Could you check a few things on this model? Use its own coordinates, in mm. Face numbers are marked on the shaded views. Give positions to 0.01 mm unless a question says otherwise; leave off trailing zeros. Order: outer loops, then holes, each group sorted by start corner. A loop starts at its lowest first (then second) coordinate and runs counter-clockwise, first axis right, second up. Notation, with made-up numbers: (82, 33) -> (109, 33) arc R21 ccw to (109, 53) -> close; hole circle Ø2 at (-30.75, -19). An arc over 180 degrees is marked (long way). One line per item, written item: value.
```python
from build123d import *

# Parameters (mm, degrees)
SKETCH1_W                      = 47.625
SKETCH1_H                      = 22.225
BOSS_EXTRUDE1_DEPTH            = 304.8
CUT_EXTRUDE1_REACH             = 27.4
SKETCH2_R                      = 14.2875
SKETCH2_R_2                    = 19.05
CUT_EXTRUDE1_DIRECTION_2_DEPTH = 1
CUT_EXTRUDE2_REACH             = 27.4
SKETCH3_R                      = 12.7
CUT_EXTRUDE2_DIRECTION_2_DEPTH = 1
SKETCH7_R                      = 4.7625
CUT_EXTRUDE3_DEPTH             = 24.8125
CUT_EXTRUDE3_DEPTH_BACK        = 2.5875
CUT_EXTRUDE4_REACH             = 27.4
SKETCH8_R                      = 3.3782
CUT_EXTRUDE4_DIRECTION_2_DEPTH = 1
CUT_EXTRUDE5_REACH             = 27.4
SKETCH9_R                      = 7.9375
CUT_EXTRUDE5_DIRECTION_2_DEPTH = 1
CUT_EXTRUDE6_REACH             = 27.4
SKETCH10_R                     = 1.5875
CUT_EXTRUDE6_DIRECTION_2_DEPTH = 1


with BuildPart() as part:
    # Sketch1 → Boss-Extrude1 (new body)
    with BuildSketch(Plane.XY):
        with BuildLine():
            Line((-23.8125, -12.7), (23.8125, -12.7))
            ThreePointArc((23.8125, -12.7), (24.935032015, -12.235032015), (25.4, -11.1125))
            Line((25.4, -11.1125), (25.4, 11.1125))
            ThreePointArc((25.4, 11.1125), (24.935032015, 12.235032015), (23.8125, 12.7))
            Line((23.8125, 12.7), (-23.8125, 12.7))
            ThreePointArc((-23.8125, 12.7), (-24.935032015, 12.235032015), (-25.4, 11.1125))
            Line((-25.4, 11.1125), (-25.4, -11.1125))
            ThreePointArc((-25.4, -11.1125), (-24.935032015, -12.235032015), (-23.8125, -12.7))
        make_face()
        Rectangle(SKETCH1_W, SKETCH1_H, mode=Mode.SUBTRACT)
    extrude(amount=BOSS_EXTRUDE1_DEPTH)

    # Sketch2 → Cut-Extrude1 (cut, up to next)
    with BuildSketch(Plane(origin=(0, 12.7, 0), x_dir=(1, 0, 0), z_dir=(0, 1, 0)), mode=Mode.PRIVATE) as cut_extrude1_sk1:
        with Locations((0, -259.9)):
            Circle(SKETCH2_R)
    cut_extrude1_tool1 = extrude(cut_extrude1_sk1.sketch, amount=-CUT_EXTRUDE1_REACH, mode=Mode.PRIVATE) & part.part
    add(cut_extrude1_tool1.solids().sort_by_distance((0, 12.7, 259.9))[0], mode=Mode.SUBTRACT)
    # Sketch2 → Cut-Extrude1 (cut, up to next)
    with BuildSketch(Plane(origin=(0, 12.7, 0), x_dir=(1, 0, 0), z_dir=(0, 1, 0)), mode=Mode.PRIVATE) as cut_extrude1_sk2:
        with Locations((0, -44.9)):
            Circle(SKETCH2_R_2)
    cut_extrude1_tool2 = extrude(cut_extrude1_sk2.sketch, amount=-CUT_EXTRUDE1_REACH, mode=Mode.PRIVATE) & part.part
    add(cut_extrude1_tool2.solids().sort_by_distance((0, 12.7, 44.9))[0], mode=Mode.SUBTRACT)

    # Sketch2 → Cut-Extrude1 direction 2 (cut)
    with BuildSketch(Plane(origin=(0, 12.7, 0), x_dir=(1, 0, 0), z_dir=(0, 1, 0))):
        with Locations((0, -259.9)):
            Circle(SKETCH2_R)
        with Locations((0, -44.9)):
            Circle(SKETCH2_R_2)
    extrude(amount=CUT_EXTRUDE1_DIRECTION_2_DEPTH, mode=Mode.SUBTRACT)

    # Sketch3 → Cut-Extrude2 (cut, up to next)
    with BuildSketch(Plane.XZ.offset(12.7), mode=Mode.PRIVATE) as cut_extrude2_sk1:
        with Locations((0, 44.9)):
            Circle(SKETCH3_R)
    cut_extrude2_tool1 = extrude(cut_extrude2_sk1.sketch, amount=-CUT_EXTRUDE2_REACH, mode=Mode.PRIVATE) & part.part
    add(cut_extrude2_tool1.solids().sort_by_distance((0, -12.7, 44.9))[0], mode=Mode.SUBTRACT)
    # Sketch3 → Cut-Extrude2 (cut, up to next)
    with BuildSketch(Plane.XZ.offset(12.7), mode=Mode.PRIVATE) as cut_extrude2_sk2:
        with Locations((0, 259.9)):
            Circle(SKETCH3_R)
    cut_extrude2_tool2 = extrude(cut_extrude2_sk2.sketch, amount=-CUT_EXTRUDE2_REACH, mode=Mode.PRIVATE) & part.part
    add(cut_extrude2_tool2.solids().sort_by_distance((0, -12.7, 259.9))[0], mode=Mode.SUBTRACT)

    # Sketch3 → Cut-Extrude2 direction 2 (cut)
    with BuildSketch(Plane.XZ.offset(12.7)):
        with Locations((0, 44.9)):
            Circle(SKETCH3_R)
        with Locations((0, 259.9)):
            Circle(SKETCH3_R)
    extrude(amount=CUT_EXTRUDE2_DIRECTION_2_DEPTH, mode=Mode.SUBTRACT)

    # Sketch7 → Cut-Extrude3 (cut, two sides)
    with BuildSketch(Plane.XZ.offset(-11.1125)) as cut_extrude3_sk:
        with Locations((17.960512242, 62.860512242)):
            Circle(SKETCH7_R)
        with Locations((-17.960512242, 26.939487758)):
            Circle(SKETCH7_R)
        with BuildLine():
            ThreePointArc((20.513212242, 26.939487758), (17.960512242, 29.492187758), (15.407812242, 26.939487758))
            ThreePointArc((15.407812242, 26.939487758), (17.960512242, 24.386787758), (20.513212242, 26.939487758))
        make_face()
        with BuildLine():
            ThreePointArc((-15.407812242, 62.860512242), (-17.960512242, 65.413212242), (-20.513212242, 62.860512242))
            ThreePointArc((-20.513212242, 62.860512242), (-17.960512242, 60.307812242), (-15.407812242, 62.860512242))
        make_face()
    extrude(amount=CUT_EXTRUDE3_DEPTH, mode=Mode.SUBTRACT)
    extrude(cut_extrude3_sk.sketch, amount=-CUT_EXTRUDE3_DEPTH_BACK, mode=Mode.SUBTRACT)

    # Sketch8 → Cut-Extrude4 (cut, up to next)
    with BuildSketch(Plane(origin=(0, 12.7, 0), x_dir=(1, 0, 0), z_dir=(0, 1, 0)), mode=Mode.PRIVATE) as cut_extrude4_sk1:
        with Locations((0, -116.566667182)):
            Circle(SKETCH8_R)
    cut_extrude4_tool1 = extrude(cut_extrude4_sk1.sketch, amount=-CUT_EXTRUDE4_REACH, mode=Mode.PRIVATE) & part.part
    add(cut_extrude4_tool1.solids().sort_by_distance((0, 12.7, 116.566667))[0], mode=Mode.SUBTRACT)
    # Sketch8 → Cut-Extrude4 (cut, up to next)
    with BuildSketch(Plane(origin=(0, 12.7, 0), x_dir=(1, 0, 0), z_dir=(0, 1, 0)), mode=Mode.PRIVATE) as cut_extrude4_sk2:
        with Locations((0, -188.233332818)):
            Circle(SKETCH8_R)
    cut_extrude4_tool2 = extrude(cut_extrude4_sk2.sketch, amount=-CUT_EXTRUDE4_REACH, mode=Mode.PRIVATE) & part.part
    add(cut_extrude4_tool2.solids().sort_by_distance((0, 12.7, 188.233333))[0], mode=Mode.SUBTRACT)

    # Sketch8 → Cut-Extrude4 direction 2 (cut)
    with BuildSketch(Plane(origin=(0, 12.7, 0), x_dir=(1, 0, 0), z_dir=(0, 1, 0))):
        with Locations((0, -116.566667182)):
            Circle(SKETCH8_R)
        with Locations((0, -188.233332818)):
            Circle(SKETCH8_R)
    extrude(amount=CUT_EXTRUDE4_DIRECTION_2_DEPTH, mode=Mode.SUBTRACT)

    # Sketch9 → Cut-Extrude5 (cut, up to next)
    with BuildSketch(Plane.XZ.offset(12.7), mode=Mode.PRIVATE) as cut_extrude5_sk1:
        with Locations((0, 116.566667182)):
            Circle(SKETCH9_R)
    cut_extrude5_tool1 = extrude(cut_extrude5_sk1.sketch, amount=-CUT_EXTRUDE5_REACH, mode=Mode.PRIVATE) & part.part
    add(cut_extrude5_tool1.solids().sort_by_distance((0, -12.7, 116.566667))[0], mode=Mode.SUBTRACT)
    # Sketch9 → Cut-Extrude5 (cut, up to next)
    with BuildSketch(Plane.XZ.offset(12.7), mode=Mode.PRIVATE) as cut_extrude5_sk2:
        with Locations((0, 188.233332818)):
            Circle(SKETCH9_R)
    cut_extrude5_tool2 = extrude(cut_extrude5_sk2.sketch, amount=-CUT_EXTRUDE5_REACH, mode=Mode.PRIVATE) & part.part
    add(cut_extrude5_tool2.solids().sort_by_distance((0, -12.7, 188.233333))[0], mode=Mode.SUBTRACT)

    # Sketch9 → Cut-Extrude5 direction 2 (cut)
    with BuildSketch(Plane.XZ.offset(12.7)):
        with Locations((0, 116.566667182)):
            Circle(SKETCH9_R)
        with Locations((0, 188.233332818)):
            Circle(SKETCH9_R)
    extrude(amount=CUT_EXTRUDE5_DIRECTION_2_DEPTH, mode=Mode.SUBTRACT)

    # Sketch10 → Cut-Extrude6 (cut, up to next)
    with BuildSketch(Plane(origin=(0, 12.7, 0), x_dir=(1, 0, 0), z_dir=(0, 1, 0)), mode=Mode.PRIVATE) as cut_extrude6_sk1:
        with Locations((17.272, -287.02)):
            Circle(SKETCH10_R)
    cut_extrude6_tool1 = extrude(cut_extrude6_sk1.sketch, amount=-CUT_EXTRUDE6_REACH, mode=Mode.PRIVATE) & part.part
    add(cut_extrude6_tool1.solids().sort_by_distance((17.272, 12.7, 287.02))[0], mode=Mode.SUBTRACT)
    # Sketch10 → Cut-Extrude6 (cut, up to next)
    with BuildSketch(Plane(origin=(0, 12.7, 0), x_dir=(1, 0, 0), z_dir=(0, 1, 0)), mode=Mode.PRIVATE) as cut_extrude6_sk2:
        with Locations((-17.272, -287.02)):
            Circle(SKETCH10_R)
    cut_extrude6_tool2 = extrude(cut_extrude6_sk2.sketch, amount=-CUT_EXTRUDE6_REACH, mode=Mode.PRIVATE) & part.part
    add(cut_extrude6_tool2.solids().sort_by_distance((-17.272, 12.7, 287.02))[0], mode=Mode.SUBTRACT)
    # Sketch10 → Cut-Extrude6 (cut, up to next)
    with BuildSketch(Plane(origin=(0, 12.7, 0), x_dir=(1, 0, 0), z_dir=(0, 1, 0)), mode=Mode.PRIVATE) as cut_extrude6_sk3:
        with Locations((0, -294.64)):
            Circle(SKETCH10_R)
    cut_extrude6_tool3 = extrude(cut_extrude6_sk3.sketch, amount=-CUT_EXTRUDE6_REACH, mode=Mode.PRIVATE) & part.part
    add(cut_extrude6_tool3.solids().sort_by_distance((0, 12.7, 294.64))[0], mode=Mode.SUBTRACT)
    # Sketch10 → Cut-Extrude6 (cut, up to next)
    with BuildSketch(Plane(origin=(0, 12.7, 0), x_dir=(1, 0, 0), z_dir=(0, 1, 0)), mode=Mode.PRIVATE) as cut_extrude6_sk4:
        with Locations((17.272, -93.922)):
            Circle(SKETCH10_R)
    cut_extrude6_tool4 = extrude(cut_extrude6_sk4.sketch, amount=-CUT_EXTRUDE6_REACH, mode=Mode.PRIVATE) & part.part
    add(cut_extrude6_tool4.solids().sort_by_distance((17.272, 12.7, 93.922))[0], mode=Mode.SUBTRACT)
    # Sketch10 → Cut-Extrude6 (cut, up to next)
    with BuildSketch(Plane(origin=(0, 12.7, 0), x_dir=(1, 0, 0), z_dir=(0, 1, 0)), mode=Mode.PRIVATE) as cut_extrude6_sk5:
        with Locations((0, -86.302)):
            Circle(SKETCH10_R)
    cut_extrude6_tool5 = extrude(cut_extrude6_sk5.sketch, amount=-CUT_EXTRUDE6_REACH, mode=Mode.PRIVATE) & part.part
    add(cut_extrude6_tool5.solids().sort_by_distance((0, 12.7, 86.302))[0], mode=Mode.SUBTRACT)
    # Sketch10 → Cut-Extrude6 (cut, up to next)
    with BuildSketch(Plane(origin=(0, 12.7, 0), x_dir=(1, 0, 0), z_dir=(0, 1, 0)), mode=Mode.PRIVATE) as cut_extrude6_sk6:
        with Locations((-17.272, -93.922)):
            Circle(SKETCH10_R)
    cut_extrude6_tool6 = extrude(cut_extrude6_sk6.sketch, amount=-CUT_EXTRUDE6_REACH, mode=Mode.PRIVATE) & part.part
    add(cut_extrude6_tool6.solids().sort_by_distance((-17.272, 12.7, 93.922))[0], mode=Mode.SUBTRACT)

    # Sketch10 → Cut-Extrude6 direction 2 (cut)
    with BuildSketch(Plane(origin=(0, 12.7, 0), x_dir=(1, 0, 0), z_dir=(0, 1, 0))):
        with Locations((17.272, -287.02)):
            Circle(SKETCH10_R)
        with Locations((-17.272, -287.02)):
            Circle(SKETCH10_R)
        with Locations((0, -294.64)):
            Circle(SKETCH10_R)
        with Locations((17.272, -93.922)):
            Circle(SKETCH10_R)
        with Locations((0, -86.302)):
            Circle(SKETCH10_R)
        with Locations((-17.272, -93.922)):
            Circle(SKETCH10_R)
    extrude(amount=CUT_EXTRUDE6_DIRECTION_2_DEPTH, mode=Mode.SUBTRACT)


solid = part.part
```
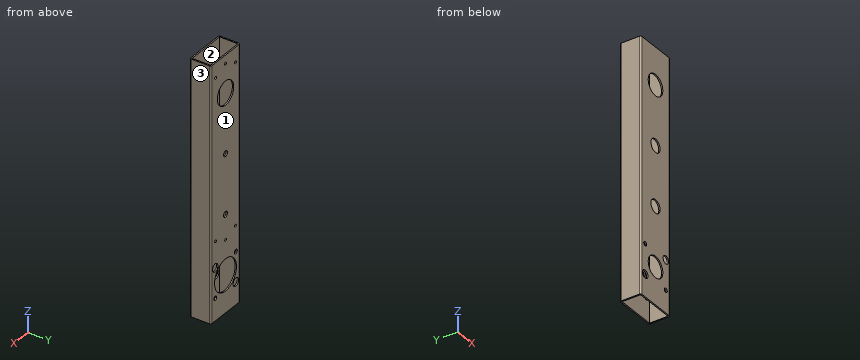
1) For P1, Ø2, axis at x = -12, y = 10, coming from the +Z side; P2, Ø3, axis at x = 0, z = 294.64, coming from the +Y side; P3, Ø14.5, axis at x = 0, z = 116.57, coming from the -Y side, each with a flat end and sliding along its axis, tell me the tip position at first contact or that it passes through.
Answer below:
P1: passes through
P2: stops at y = -11.11
P3: stops at y = 11.11
2) Suppose I cut it at A-A, the plane z = 81. Write out the boundary of the cut face in (x, y) (1 decimal).
Answer below:
outline: (-25.4, -11.1) arc R1.6 ccw to (-23.8, -12.7) -> (23.8, -12.7) arc R1.6 ccw to (25.4, -11.1) -> (25.4, 11.1) arc R1.6 ccw to (23.8, 12.7) -> (-23.8, 12.7) arc R1.6 ccw to (-25.4, 11.1) -> close; hole (-23.8, -11.1) -> (23.8, -11.1) -> (23.8, 11.1) -> (-23.8, 11.1) -> close
3) Suppose I cut it at B-B, the plane y = -8. Write out the boundary of the cut face in (x, z).
Answer below:
outline: (-25.4, 0) -> (-23.81, 0) -> (-23.81, 304.8) -> (-25.4, 304.8) -> close; (23.81, 0) -> (25.4, 0) -> (25.4, 304.8) -> (23.81, 304.8) -> close
4) If I drill on line 1 along Z through (x, y) = (0, -12); line 2 along X through (y, z) = (11.5, 287.02); line 3 along X through (y, z) = (9.25, 98), over which ranges is the centre line in solid material (lowest first)?
Answer below:
line 1: z = 0 to 32.2, 57.6 to 108.63, 124.5 to 180.3, 196.17 to 247.2, 272.6 to 304.8
line 2: x = -25.35 to -18.86, -15.68 to 15.68, 18.86 to 25.35
line 3: x = -25.4 to -23.81, 23.81 to 25.4
5) We'd pull the mould along X, two halves only. Please class the marked faces 1, 2 and 3: +X half, -X half, draft (parallel to the pull), parting line (faces both ways), or undercut.
Answer below:
face 1: draft
face 2: undercut
face 3: +X half
